Geometry: final body of the model. Coordinates: model frame, mm. A direction names the side the tool comes from. Give positions to 0.01 mm unless a question says otherwise; leave off trailing zeros. Order: outer loops, then holes, each group sorted by start corner. A loop starts at its lowest first (then second) coordinate and runs counter-clockwise, first axis right, second up. Notation, with made-up numbers: (4.5, 19) -> (47.5, 19) arc R16 ccw to (47.5, 27) -> close; hole circle Ø11 at (57, 3.25). An arc over 180 degrees is marked (long way). One line per question, with ' | ' between items. Start each with the question number.
(1) Section C-C (y = 347.5). Return loops of the section in (x, z).
(2) Section B-B (z = 0). Return loops of the section in (x, y), then the cut area to 3 significant figures.
(3) Mould query, pull axis X, two halves, no side actions, for faces 4 (the face through (4, -10, -255)), 5 (the face through (-3, 2, 215)), 6 (the face through (-250, 2, -27)). Classes: +X half, -X half, draft (parallel to the pull), parting line (faces both ways), or undercut.
(4) First-contact query: pin 1 Ø3 at (x, z) = (-143, 11) entering from -Y; pin 2 Ø3 at (x, z) = (32, 222) entering from +Y; pin 3 Ø11 at (x, z) = (71, -237.5) entering from +Y. Flat tips, straight axial feed; report the tip coordinate or a pass-through.
(5) Ray query, L1, parallel to Z at x = 2, y = -125; L2, parallel to X at y = -128, z = 0; L3, parallel to Y at x = -20.5, z = -73. Return the intervals inside material, ascending.
(6) Set-up query: faces 1 (the face through (3.08, -190.979, 216.445)), 2 (the face through (173.51, 347.9, -22.78)), 3 (the face through (2, 0, 2)). Return all of +Z, -Z, +X, -X, +Y, -Y with unobstructed straight access to the full face (end or side cutting, diameter ignored); none if empty.
(7) Section D-D (z = 183.5). Return loops of the section in (x, y), then the cut area to 3 significant figures.
(8) Section A-A (y = -64). Return loops of the section in (x, z), then the cut area to 3 significant figures.
```python
from build123d import *

# Parameters (mm, degrees)
SKETCH1_W           = 500
SKETCH1_H           = 450
BOSS_EXTRUDE1_DEPTH = 200
BOSS_EXTRUDE2_DEPTH = 500
FILLET1_R           = 5
SKETCH3_R           = 150
CUT_EXTRUDE1_DEPTH  = 200
SKETCH4_R           = 175
BOSS_EXTRUDE3_DEPTH = 350
FILLET2_R           = 50
FILLET3_R           = 30
SKETCH5_W           = 400
SKETCH5_H           = 300
CUT_EXTRUDE2_DEPTH  = 10


with BuildPart() as part:
    # Sketch1 → Boss-Extrude1 (new, symmetric)
    with BuildSketch(Plane(origin=(0, 0, 0), x_dir=(1, 0, 0), z_dir=(0, 1, 0))):
        Rectangle(SKETCH1_W, SKETCH1_H)
    extrude(amount=BOSS_EXTRUDE1_DEPTH, both=True)

    # Sketch2 → Boss-Extrude2 (add)
    with BuildSketch(Plane(origin=(250, 0, 0), x_dir=(0, 0, -1), z_dir=(1, 0, 0))):
        Polygon((240, -27.5), (255, -42.5), (255, 22.5), (240, 7.5), (225, 7.5), (225, -27.5), align=None)
        Polygon((225, -147.5), (225, -112.5), (240, -112.5), (255, -97.5), (255, -162.5), (240, -147.5), align=None)
    extrude(amount=-BOSS_EXTRUDE2_DEPTH)

    # Fillet1
    fillet1_edges = [part.edges().sort_by_distance(p)[0] for p in [
        (0, -147.5, -225),
        (0, -112.5, -225),
        (0, -97.5, -255),
        (0, -162.5, -255),
        (0, -27.5, -225),
        (0, 7.5, -225),
        (0, 22.5, -255),
        (0, -42.5, -255),
    ]]
    fillet(fillet1_edges, radius=FILLET1_R)

    # Sketch3 → Cut-Extrude1 (cut)
    with BuildSketch(Plane.XZ.offset(200)):
        with Locations(Location((0, 0, 0), (0, 0, 270))):
            Circle(SKETCH3_R)
    extrude(amount=-CUT_EXTRUDE1_DEPTH, mode=Mode.SUBTRACT)

    # Sketch4 → Boss-Extrude3 (add)
    with BuildSketch(Plane(origin=(0, 200, 0), x_dir=(1, 0, 0), z_dir=(0, 1, 0))):
        with Locations(Location((0, 0, 0), (0, 0, 270))):
            Circle(SKETCH4_R)
    extrude(amount=BOSS_EXTRUDE3_DEPTH)

    # Fillet2
    fillet2_edges = [part.edges().sort_by_distance(p)[0] for p in [
        (0, 550, -175),
    ]]
    fillet(fillet2_edges, radius=FILLET2_R)

    # Fillet3
    fillet3_edges = [part.edges().sort_by_distance(p)[0] for p in [
        (-250, 200, 0),
        (0, 200, 225),
        (250, 200, 0),
        (0, -200, 225),
        (-250, -200, 0),
        (250, -200, 0),
        (250, 0, 225),
        (-250, 0, 225),
    ]]
    fillet(fillet3_edges, radius=FILLET3_R)

    # Sketch5 → Cut-Extrude2 (cut)
    with BuildSketch(Plane.XY.offset(225)):
        Rectangle(SKETCH5_W, SKETCH5_H)
    extrude(amount=-CUT_EXTRUDE2_DEPTH, mode=Mode.SUBTRACT)


solid = part.part
```
Response:
1) outline: circle Ø350 at (0, 0)
2) outline: (-250, -170) arc R30 ccw to (-220, -200) -> (-150, -200) -> (-150, 0) -> (150, 0) -> (150, -200) -> (220, -200) arc R30 ccw to (250, -170) -> (250, 170) arc R30 ccw to (220, 200) -> (175, 200) -> (175, 500) arc R50 ccw to (125, 550) -> (-125, 550) arc R50 ccw to (-175, 500) -> (-175, 200) -> (-220, 200) arc R30 ccw to (-250, 170) -> close | area: 261,000 mm^2
3) face 4: draft | face 5: undercut | face 6: -X half
4) pin 1: stops at y = 0 | pin 2: stops at y = 185.8 | pin 3: stops at y = 10.5
5) L1: z = -255 to -149.99, 149.99 to 215 | L2: x = -250 to -150, 150 to 250 | L3: y = 0 to 550
6) face 1: +Z, +X, -X, -Y | face 2: +Y | face 3: -Y
7) outline: (-250, -170) arc R30 ccw to (-220, -200) -> (220, -200) arc R30 ccw to (250, -170) -> (250, 170) arc R30 ccw to (220, 200) -> (-220, 200) arc R30 ccw to (-250, 170) -> close | area: 199,000 mm^2
8) outline: (-250, -225) -> (250, -225) -> (250, 195) arc R30 ccw to (220, 225) -> (200, 225) -> (200, 215) -> (-200, 215) -> (-200, 225) -> (-220, 225) arc R30 ccw to (-250, 195) -> close; hole circle Ø300 at (0, 0) | area: 150,000 mm^2
